Verification items for the finished model (mm, model axes). A direction names the side the tool comes from. Give positions to 0.01 mm unless a question says otherwise; leave off trailing zeros. Loops run counter-clockwise (first coordinate to the right, second up) from the corner with the lowest first, then second, coordinate; pieces in that order, holes last. Notation, with made-up numbers: (32, 17) - (51, 17) arc R7 ccw to (51, 21) - close; hole circle Ø1 at (-37, 53.5). An arc over 180 degrees is marked (long way). Use one line per item in the form item = value.
```python
from build123d import *

# Parameters (mm, degrees)
F1_DEPTH = 25
F2_R     = 1.558197
F2_R_2   = 1.810611
F3_DEPTH = 25
F4_R     = 1.495771
F5_DEPTH = 25
F6_R     = 2


with BuildPart() as f1:
    # F0 (on Front) → F1 (new body)
    with BuildSketch(Plane.XZ):
        with BuildLine():
            Line((-43.781251, -2.71875), (-43.781251, -6.281251))
            Line((-43.781251, -6.281251), (-25.156251, -6.281251))
            ThreePointArc((-25.156251, -6.281251), (-21.620717, -4.816785), (-20.156251, -1.281251))
            Line((-20.156251, -1.281251), (-20.156251, -1.15625))
            ThreePointArc((-20.156251, -1.15625), (-18.691785, 2.379284), (-15.156251, 3.84375))
            Line((-15.156251, 3.84375), (2.906251, 3.84375))
            Line((2.906251, 3.84375), (2.906251, 8.906251))
            Line((2.906251, 8.906251), (-20.406251, 8.906251))
            ThreePointArc((-20.406251, 8.906251), (-23.941785, 7.441785), (-25.406251, 3.906251))
            Line((-25.406251, 3.906251), (-25.406251, 2.28125))
            ThreePointArc((-25.406251, 2.28125), (-26.870717, -1.254284), (-30.406251, -2.71875))
            Line((-30.406251, -2.71875), (-43.781251, -2.71875))
        make_face()
    extrude(amount=F1_DEPTH)

    # F2 (on face) → F3 (cut)
    with BuildSketch(Plane.XY.offset(-2.71875)):
        with Locations((-39.640795, -4.70578)):
            Circle(F2_R)
        with Locations((-39.078295, -20.455781)):
            Circle(F2_R_2)
    extrude(amount=-F3_DEPTH, mode=Mode.SUBTRACT)

    # F4 (on face) → F5 (cut)
    with BuildSketch(Plane.XY.offset(8.906251)):
        with BuildLine():
            ThreePointArc((-0.577267, -5.833911), (1.942488, -7.647325), (2.906251, -10.598393))
            Line((2.906251, -10.598393), (2.906251, 0))
            Line((2.906251, 0), (-18.906251, 0))
            Line((-18.906251, 0), (-0.577267, -5.833911))
        make_face()
        with BuildLine():
            Line((2.906251, -25), (2.906251, -13.569611))
            ThreePointArc((2.906251, -13.569611), (2.001345, -16.438445), (-0.385832, -18.268869))
            Line((-0.385832, -18.268869), (-18.906251, -25))
            Line((-18.906251, -25), (2.906251, -25))
        make_face()
        with Locations((-16.0868, -12.426148)):
            Circle(F4_R)
        with BuildLine():
            ThreePointArc((-4.555258, -10.445567), (-7.775122, -11.030102), (-11.047432, -10.995579))
            ThreePointArc((-11.047432, -10.995579), (-12.632527, -12.304577), (-11.29052, -13.861825))
            Line((-11.29052, -13.861825), (-11.275081, -13.867438))
            ThreePointArc((-11.275081, -13.867438), (-7.493954, -13.896562), (-3.774169, -13.217624))
            Line((-3.774169, -13.217624), (-3.747407, -13.206846))
            ThreePointArc((-3.747407, -13.206846), (-2.784389, -11.426288), (-4.555258, -10.445567))
        make_face()
    extrude(amount=-F5_DEPTH, mode=Mode.SUBTRACT)

    # F6
    f6_edges = [f1.edges().sort_by_distance(p)[0] for p in [
        (-43.781251, 0, -4.5),
        (-43.781251, -25, -4.5),
    ]]
    fillet(f6_edges, radius=F6_R)


solid = f1.part
```
1. Tool access check on faces 1 (the flat face through (-25.406, -12, 3)), 2 (the flat face through (-25, 0, 0)), 3 (the cylindrical face through (-12.63, -12.27, 6.41)). Record the directions out of +Z, -Z, +X, -X, +Y, -Y that give a thin tool (end or side, any length) a straight path to the whole face; none if there is none.
Result set:
face_1 = +Z, -X, +Y, -Y
face_2 = +Z, -Z, +X, -X, +Y
face_3 = +Z, -Z
2. Depth check by flat-ended pin: pin 1 Ø8 at (x, y) = (-11, -9.5) entering from -Z; pin 2 Ø14.5 at (x, y) = (-36, -13) entering from +Z; pin 3 Ø2 at (x, z) = (-3, 3.5) entering from +Y. Enter the tip coordinate at first touch or a pass-through.
Result set:
pin_1 = 3.84
pin_2 = -2.44
pin_3 = -4.76
3. Section check C-C, the plane x = -5.5. Record the cut outline in (y, z).
Result set:
outline = (-20.13, 3.84) - (-13.62, 3.84) - (-13.62, 8.91) - (-20.13, 8.91) - close; (-10.68, 3.84) - (-4.27, 3.84) - (-4.27, 8.91) - (-10.68, 8.91) - close
4. Scan lines: probe 1 along Z at (x, y) = (-3.5, -10); probe 2 along X at (y, z) = (-4.75, 2.75); probe 3 along Z at (x, y) = (-34, -22.25). Record each from-to range of solid material in increasing order.
Result set:
probe_1 = 3.84 to 8.91
probe_2 = -25.41 to -18.28
probe_3 = -6.28 to -2.72
5. Section check B-B, the plane z = -3.5. Record the cut outline in (x, y).
Result set:
outline = (-43.78, -23) arc R2 ccw to (-41.78, -25) - (-20.68, -25) - (-20.68, 0) - (-41.78, 0) arc R2 ccw to (-43.78, -2) - close; hole circle Ø3.12 at (-39.64, -4.71); hole circle Ø3.62 at (-39.08, -20.46)
6. Draft check along X on faces 4 (the cylindrical face through (-7.729, -11.026, 6.41)), 5 (the flat face through (-43.781, -12, -4)), 6 (the cylindrical face through (1.916, -7.612, 6.41)). Enter one of: released by +X, released by -X, zero draft, split by the parting line, or undercut.
Result set:
face_4 = undercut
face_5 = released by -X
face_6 = released by +X
7. Section check A-A, the plane y = -4.25. Record the cut outline in (x, z), then the cut area to 3 significant figures.
Result set:
outline = (-43.78, -6.28) - (-41.13, -6.28) - (-41.13, -2.72) - (-43.78, -2.72) - close; (-38.15, -6.28) - (-25.16, -6.28) arc R5 ccw to (-20.16, -1.28) - (-20.16, -1.16) arc R5 cw to (-15.16, 3.84) - (-5.55, 3.84) - (-5.55, 8.91) - (-20.41, 8.91) arc R5 ccw to (-25.41, 3.91) - (-25.41, 2.28) arc R5 cw to (-30.41, -2.72) - (-38.15, -2.72) - close
area = 209 mm²
8. Section check D-D, the plane y = -11.75. Record the cut outline in (x, z), then the cut area to 3 significant figures.
Result set:
outline = (-43.78, -6.28) - (-25.16, -6.28) arc R5 ccw to (-20.16, -1.28) - (-20.16, -1.16) arc R5 cw to (-17.42, 3.3) - (-17.42, 8.91) - (-20.41, 8.91) arc R5 ccw to (-25.41, 3.91) - (-25.41, 2.28) arc R5 cw to (-30.41, -2.72) - (-43.78, -2.72) - close; (-14.75, 3.84) - (-12.47, 3.84) - (-12.47, 8.91) - (-14.75, 8.91) - close; (-2.73, 3.84) - (2.91, 3.84) - (2.91, 8.91) - (-2.73, 8.91) - close
area = 199 mm²
